Read the model definition and answer for the solid it produces. Units are mm, in the model's axes. A direction names the side the tool comes from. Round coordinates to 2 decimals unless told otherwise and drop trailing zeros. Order: outer loops, then holes, each group sorted by start corner. A loop starts at its lowest first (then second) coordinate and runs counter-clockwise, first axis right, second up. Notation, with made-up numbers: M 78,39 L 87,39 A19 ccw 87,65 Z; hole C 13.25,20.25 d10. An arc over 180 degrees is marked long. Answer as CSV lines item,"result".
Autodesk Inventor part; units mm, degrees
ref_plane "YZ Plane" through (0, 0, 0) normal (1, 0, 0) x (0, 1, 0)
ref_plane "XZ Plane" through (0, 0, 0) normal (0, 1, 0) x (-1, 0, 0)
ref_plane "XY Plane" through (0, 0, 0) normal (0, 0, 1) x (1, 0, 0)
ref_plane "boardTop(tolerance)" through (29.1257, 19.6924, 40.7272) normal (0, -1, 0) x (1, 0, 0)
sketch "Sketch3" plane through (29.1257, 19.6924, 40.7272) normal (0, -1, 0) x (1, 0, 0)
  line L0 (-2, 1.51) -> (-2, 0)
  line L1 (158.35, 0) -> (158.35, 1.51)
  line L2 (-11, 18.0177) -> (-11, -5)
  line L3 (167.35, 18.0177) -> (167.35, -5)
  line L4 (167.35, 18.0177) -> (-11, 18.0177)
  line L5 (-11, -5) -> (167.35, -5)
  point P0 (-29.1257, -40.7272)
  point P1 (158.35, 0.755)
  dimension "d12" = 9
  dimension "d13" = 9
extrude "Extrusion3" add sketch "Sketch3" against normal blind 5
ref_plane "boardBottom(tolerance)" through (185.4757, -59.8376, 42.2372) normal (0, -1, 0) x (-1, 0, 0)
sketch "Sketch4" plane through (29.1257, 19.6924, 40.7272) normal (0, -1, 0) x (1, 0, 0)
  line L0 (-2, 1.51) -> (-2, 0)
  line L1 (158.35, 1.51) -> (158.35, 0)
  line L2 (-11, 18.0177) -> (-11, -5)
  line L3 (-11, -5) -> (167.35, -5)
  line L4 (167.35, -5) -> (167.35, 18.0177)
  line L5 (167.35, 18.0177) -> (-11, 18.0177)
  line L6 (159.35, -5) -> (159.35, 18.0177)
  line L7 (-11, 18.0177) -> (167.35, 18.0177)
  line L8 (-3, -5) -> (-3, 18.0177)
  point P0 (-29.1257, -40.7272)
  point P1 (158.35, 0.755)
  point P2 (-2, 0.755)
  point P3 (-3, 18.0177)
  dimension "d17" = 1
  dimension "d18" = 1
extrude "Extrusion4" add sketch "Sketch4" along normal blind 94.5274 contours L5 L8 L3 L2 | L5 L4 L3 L6
ref_plane "boardRight(tolerance)" through (188.4757, 19.6924, 35.7272) normal (-1, 0, 0) x (0, -1, 0)
sketch "Sketch5" plane through (188.4757, -74.835, 35.7272) normal (-1, 0, 0) x (0, 0, 1)
  line L0 (5, 15.9974) -> (6.51, 15.9974)
  line L1 (0, 94.5274) -> (23.0177, 94.5274)
  line L2 (0, 94.5274) -> (0, 0)
  line L3 (23.0177, 0) -> (0, 0)
  line L4 (23.0177, 94.5274) -> (23.0177, 0)
  line L5 (0, 94.5274) -> (0, 0)
  line L6 (0, 15.9974) -> (23.0177, 15.9974)
  line L7 (23.0177, 15.9974) -> (23.0177, 12.9974)
  line L8 (23.0177, 12.9974) -> (0, 12.9974)
  line L9 (0, 12.9974) -> (0, 15.9974)
  point P0 (-35.7272, 74.835)
  point P1 (0, 12.9974)
  point P2 (6.51, 15.9974)
  dimension "d21" = 3
ref_plane "boardLeft(tolerance)" through (26.1257, 19.6924, 58.7449) normal (1, 0, 0) x (0, -1, 0)
extrude "Extrusion5" add sketch "Sketch5" along normal up to surface (162.35 mm away) contours L0 L6 L4 L8 L2
sketch "Sketch6" plane through (29.1257, 19.6924, 40.7272) normal (0, -1, 0) x (1, 0, 0)
  line L0 (48.3131, 6.295) -> (48.54, 4.395)
  line L1 (54.3069, 2.495) -> (54.08, 4.395)
  line L2 (99.8531, 6.295) -> (100.08, 4.395)
  line L3 (107.5969, 2.495) -> (107.37, 4.395)
  line L4 (-3, 18.0177) -> (-3, -5)
  line L5 (-3, -5) -> (159.35, -5)
  line L6 (159.35, -5) -> (159.35, 18.0177)
  line L7 (159.35, 18.0177) -> (-3, 18.0177)
  line L8 (0, 1.51) -> (156.35, 1.51)
  line L9 (102.725, 1.51) -> (104.725, 1.51)
  line L10 (104.725, 1.51) -> (104.725, 18.0177)
  line L11 (104.725, 18.0177) -> (102.725, 18.0177)
  line L12 (102.725, 18.0177) -> (102.725, 1.51)
  line L13 (159.35, 18.0177) -> (-3, 18.0177)
  line L14 (50.31, 1.51) -> (52.31, 1.51)
  line L15 (52.31, 1.51) -> (52.31, 18.0177)
  line L16 (52.31, 18.0177) -> (50.31, 18.0177)
  line L17 (50.31, 18.0177) -> (50.31, 1.51)
  line L18 (48.4266, 5.345) -> (50.31, 5.345) construction
  line L19 (54.1934, 3.445) -> (52.31, 3.445) construction
  line L20 (99.9666, 5.345) -> (102.725, 5.345) construction
  line L21 (107.4834, 3.445) -> (104.725, 3.445) construction
  point P0 (-29.1257, -40.7272)
  point P1 (124.6421, 15.795)
  dimension "d31" = 2
  dimension "d32" = 2
extrude "Extrusion6" add sketch "Sketch6" along normal blind 44.45 contours L7 L15 L8 L17 | L7 L10 L8 L12
sketch "Sketch7" plane through (133.8507, 19.6924, 42.2372) normal (0, 0, -1) x (-1, 0, 0)
  line L0 (2, 0) -> (2, -44.45)
  line L1 (0, 0) -> (0, -44.45)
  line L2 (2, -44.45) -> (0, -44.45)
  line L3 (54.415, 0) -> (54.415, -44.45)
  line L4 (52.415, 0) -> (52.415, -44.45)
  line L5 (54.415, -44.45) -> (52.415, -44.45)
  line L6 (0, 0) -> (2, 0)
  line L7 (54.415, 0) -> (52.415, 0)
  point P0 (133.8507, -19.6924)
extrude "Extrusion7" cut sketch "Sketch7" against normal blind 3
sketch "Sketch9" plane through (188.4757, 19.6924, 35.7272) normal (-1, 0, 0) x (0, 0, 1)
  line L0 (9.51, -38.275) -> (23.0177, -38.275)
  line L1 (9.51, -36.275) -> (23.0177, -36.275)
  line L2 (9.51, -36.275) -> (23.0177, -36.275)
  line L3 (23.0177, -36.275) -> (23.0177, -38.275)
  line L4 (23.0177, -38.275) -> (9.51, -38.275)
  line L5 (9.51, -38.275) -> (9.51, -36.275)
  point P0 (-35.7272, -19.6924)
  dimension "d37" = 2
extrude "Extrusion8" add sketch "Sketch9" along normal up to surface (162.35 mm away)
fillet "Fillet1" radius 4.7625 2 edges at (18.1257, 24.6924, 47.236) (196.4757, 24.6924, 47.236)
sketch "Sketch10" plane through (196.4757, 19.6924, 35.7272) normal (-1, 0, 0) x (0, 0, 1)
  line L0 (10.3897, -67.2551) -> (10.3897, -61.4051)
  line L1 (7.715, -63.9401) -> (7.715, -66.58)
  line L2 (9.495, -60.3354) -> (8.9571, -60.3354)
  line L3 (8.9571, -68.3248) -> (9.495, -68.3248)
  arc A0 (10.145, -61.0301) -> (9.695, -60.5801) centre (9.695, -61.0301) ccw
  line L4 (8.4889, -60.7119) -> (7.8268, -61.374)
  line L5 (7.8268, -67.2862) -> (8.4889, -67.9483)
  line L6 (7.715, -62.0803) -> (7.715, -63.9301)
  line L7 (7.715, -63.9401) -> (7.715, -66.58)
  line L8 (10.3897, -67.2551) -> (10.3897, -61.4051)
  line L9 (11.2274, -71.6801) -> (6.8774, -71.6801)
  line L10 (4.8774, -69.6801) -> (4.8774, -58.9801)
  line L11 (6.8774, -56.9801) -> (11.2274, -56.9801)
  line L12 (13.2274, -58.9801) -> (13.2274, -69.6801)
  line L13 (9.226, -68.3248) -> (9.2261, -71.6801) construction
  line L14 (9.226, -60.3354) -> (9.226, -56.9801) construction
  line L15 (13.2274, -64.3301) -> (10.3897, -64.3301) construction
  line L16 (7.715, -64.3301) -> (4.8774, -64.3301) construction
  arc A1 (13.2274, -58.9801) -> (11.2274, -56.9801) centre (11.2274, -58.9801) ccw
  arc A2 (6.8774, -56.9801) -> (4.8774, -58.9801) centre (6.8774, -58.9801) ccw
  arc A3 (4.8774, -69.6801) -> (6.8774, -71.6801) centre (6.8774, -69.6801) ccw
  arc A4 (11.2274, -71.6801) -> (13.2274, -69.6801) centre (11.2274, -69.6801) ccw
  point P0 (-35.7272, -19.6924)
  point P1 (7.685, -61.1849)
  point P2 (13.2274, -71.6801)
  point P3 (4.8774, -56.9801)
  point P4 (4.8774, -71.6801)
  point P5 (13.2274, -56.9801)
  point P6 (9.495, -68.3248)
  dimension "d47" = 8.35
  dimension "d48" = 14.7
  dimension "d49" = 2
extrude "Extrusion9" cut sketch "Sketch10" along normal blind 8
sketch "Sketch11" plane through (196.4757, -74.835, 35.7272) normal (0, 0, -1) x (-1, 0, 0)
  arc A0 (4.7625, 99.5274) -> (0, 94.7649) centre (4.7625, 94.7649) ccw
  line L0 (0, 94.7649) -> (0, 0)
  line L1 (8, 0) -> (0, 0)
  line L2 (8, 12.9974) -> (8, 0)
  line L3 (8, 12.9974) -> (170.35, 12.9974)
  line L4 (170.35, 12.9974) -> (170.35, 0)
  line L5 (178.35, 0) -> (170.35, 0)
  line L6 (178.35, 94.7649) -> (178.35, 0)
  arc A1 (178.35, 94.7649) -> (173.5875, 99.5274) centre (173.5875, 94.7649) ccw
  line L7 (4.7625, 99.5274) -> (173.5875, 99.5274)
  line L8 (8, 15.9974) -> (170.35, 15.9974)
  line L9 (8, 94.5274) -> (8, 15.9974)
  line L10 (170.35, 94.5274) -> (8, 94.5274)
  line L11 (170.35, 94.5274) -> (170.35, 15.9974)
  point P0 (196.4757, 74.835)
extrude "Extrusion10" add sketch "Sketch11" along normal blind 5
properties part number "case"
Item 1: Find the intervals of material crossed by probe 1 along Y at (x, z) = (87, 55.5); probe 2 along X at (y, z) = (1, 49.5); probe 3 along X at (y, z) = (-68, 54), in increasing order. Write a range as [from, to].
Ans:
probe 1,"[-61.84, -58.84], [-18.58, -16.58], [19.69, 24.69]"
probe 2,"[18.13, 26.13], [79.44, 81.44], [131.85, 133.85], [188.48, 196.48]"
probe 3,"[18.13, 26.13], [188.48, 196.48]"
Item 2: Determine the mould class of faces 1 (the face through (18.126, -27, 45)), 2 (the face through (193, -51.988, 45)), 3 (the face through (108, -18, 58.745)) for opening direction Z: +Z half, -Z half, draft (parallel to the pull), parting line (faces both ways), or undercut.
Ans:
face 1,"draft"
face 2,"undercut"
face 3,"+Z half"
Item 3: Flat-ended cylindrical pins translate along their axes: pin 1 (4 mm diameter, centred on x = 166.5, z = 51, fed in from -Y); pin 2 (1 mm diameter, centred on x = 78.5, y = 12.5, fed in from -Z); pin 3 (22 mm diameter, centred on x = 145, y = -11.5, fed in from -Z). Find the tip coordinate at first contact, or state that the pin passes through.
Ans:
pin 1,"y = -61.84"
pin 2,"through"
pin 3,"z = 45.24"
Item 4: A cutting plane is placed at C-C, the plane y = -21. Determine the outline of the cut face in (x, z).
Ans:
outline,"M 18.13,30.73 L 26.13,30.73 L 26.13,58.74 L 18.13,58.74 Z; M 79.44,45.24 L 81.44,45.24 L 81.44,58.74 L 79.44,58.74 Z; M 131.85,45.24 L 133.85,45.24 L 133.85,58.74 L 131.85,58.74 Z; M 188.48,30.73 L 196.48,30.73 L 196.48,58.74 L 188.48,58.74 Z"
Item 5: A tool of negligible diameter and unlimited length cuts with its end or side. For faces 4 (the face through (108, -17, 45.237)), 5 (the face through (81.436, -22, 52)), 6 (the face through (193, -37.288, 45)), from which of +Z, -Z, +X, -X, +Y, -Y can it reach the whole face along a straight path? Write none if from no direction.
Ans:
face 4,"-Z"
face 5,"+Z, -Z"
face 6,"+X"
Item 6: A cutting plane is placed at B-B, the plane z = 34.5. Determine the outline of the cut face in (x, y) (1 decimal).
Ans:
outline,"M 18.1,-74.8 L 26.1,-74.8 L 26.1,-61.8 L 188.5,-61.8 L 188.5,-74.8 L 196.5,-74.8 L 196.5,19.9 A4.8 ccw 191.7,24.7 L 22.9,24.7 A4.8 ccw 18.1,19.9 Z; hole M 26.1,-58.8 L 188.5,-58.8 L 188.5,19.7 L 26.1,19.7 Z"
Item 7: A cutting plane is placed at D-D, the plane z = 57. Give the number of separate pieces and of enclosed holes in the cut face, and give its area (3 significant figures).
Ans:
separate pieces,"1"
enclosed holes,"4"
area,"3,380 mm2"
Item 8: A cutting plane is placed at A-A, the plane x = 56. Determine the outline of the cut face in (y, z), and give its area (3 significant figures).
Ans:
outline,"M -61.84,30.73 L -58.84,30.73 L -58.84,58.74 L -61.84,58.74 Z; M -18.58,45.24 L -16.58,45.24 L -16.58,58.74 L -18.58,58.74 Z; M 19.69,30.73 L 24.69,30.73 L 24.69,58.74 L 19.69,58.74 Z"
area,"251 mm2"
